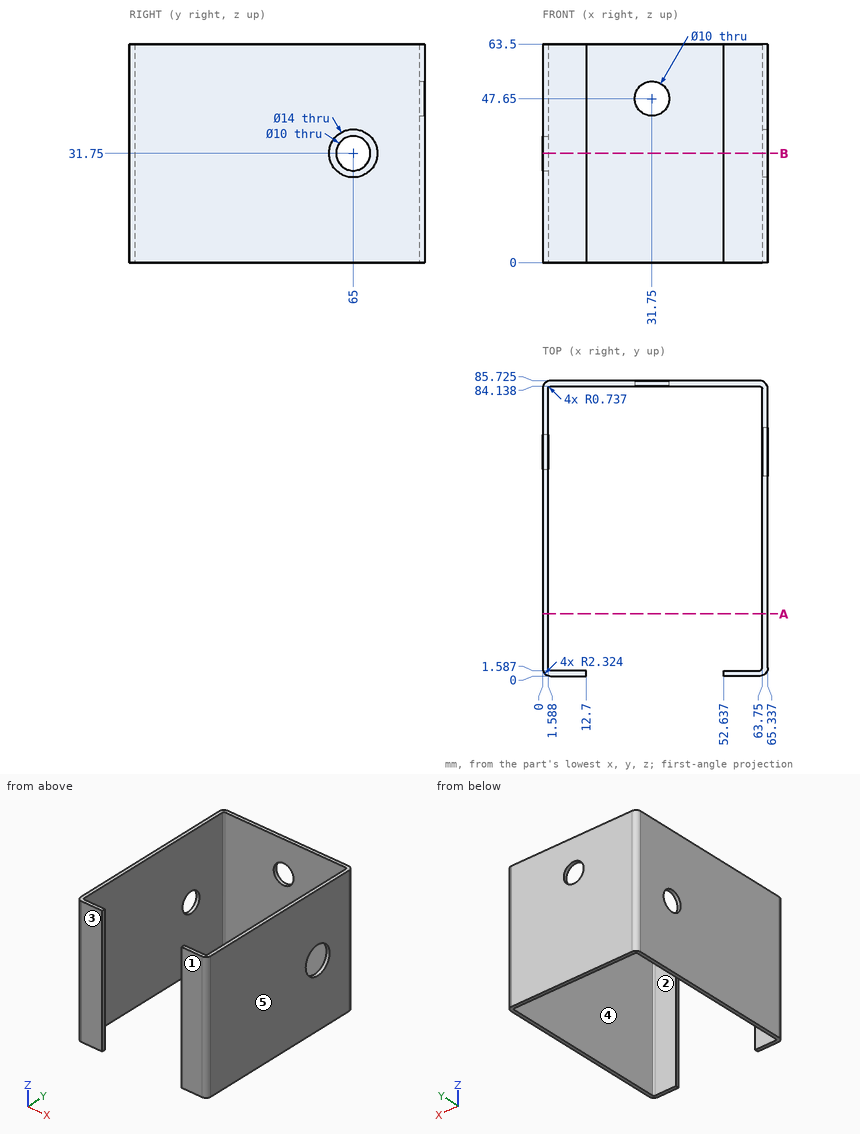
Input: dimensioned drawing with shaded views. Units: mm. Origin: part minimum x, y, z. A direction names the side the tool comes from. Coordinates: 2 decimals unless noted, no trailing zeros. Loops run counter-clockwise (first coordinate to the right, second up) from the corner with the lowest first, then second, coordinate; pieces in that order, holes last. Notation, with made-up numbers: (66.5, -13.5) -> (91.5, -13.5) arc R7 cw to (91.5, -1.5) -> close; hole circle Ø2 at (29, 61.25). An arc over 180 degrees is marked (long way). Use a Markdown table: item, result. Add a question column.
(1) Line query: line 1 along X through (y, z) = (11.5, 53.5); line 2 along Y through (x, z) = (59, 15.5) (1 decimal); line 3 along Y through (x, z) = (40.5, 19) (1 decimal). Output: solid intervals per line, ascending.
(2) Section query B-B, the plane z = 31.75. State how many separate pieces and enclosed holes the cut face has.
(3) Section query A-A, the plane y = 18. Return loops of the section in (x, z).
(4) Pin query (flat end, axial travel): pin 1 Ø2 at (x, z) = (51, 33.5) entering from -Y; pin 2 Ø0.8 at (y, z) = (0.5, 19.5) entering from +X; pin 3 Ø1.3 at (y, z) = (0.5, 27) entering from -X. Return the tip coordinate at first contact, or that it passes through.
(5) Access query for the marked faces 1 and 2. Directions: +Z, -Z, +X, -X, +Y, -Y. A direction counts if a zero-diameter tool reaches every point of the face in a straight line with its end or side. Return the directions, or none.
(6) Mould query, pull axis Y, two halves, no side actions, for the marked faces 3, 4 and 5. Classes: pulls with the +Y half, pulls with the -Y half, needs draft (parallel to the pull), parting line crosses it, or undercut.
Answer:
| question | item | result |
|---|---|---|
| 1 | line 1 | x = 0 to 1.59, 63.75 to 65.34 |
| 1 | line 2 | y = 0 to 1.6, 84.1 to 85.7 |
| 1 | line 3 | y = 84.1 to 85.7 |
| 2 | separate pieces | 3 |
| 2 | enclosed holes | 0 |
| 3 | outline | (0, 0) -> (1.59, 0) -> (1.59, 63.5) -> (0, 63.5) -> close; (63.75, 0) -> (65.34, 0) -> (65.34, 63.5) -> (63.75, 63.5) -> close |
| 4 | pin 1 | stops at y = 84.14 |
| 4 | pin 2 | stops at x = 64.85 |
| 4 | pin 3 | stops at x = 0.32 |
| 5 | face 1 | +Z, -Z, +X, -X, -Y |
| 5 | face 2 | +Z, -Z |
| 6 | face 3 | pulls with the -Y half |
| 6 | face 4 | undercut |
| 6 | face 5 | needs draft |
